Verification items for the finished model (mm, model axes). Face numbers are marked on the shaded views. A direction names the side the tool comes from. Give positions to 0.01 mm unless a question says otherwise; leave off trailing zeros. Write each loop counter-clockwise with the first axis right and the second up, starting at its lowest first coordinate (ties: lowest second). Pieces come first, ordered by that corner, then holes.
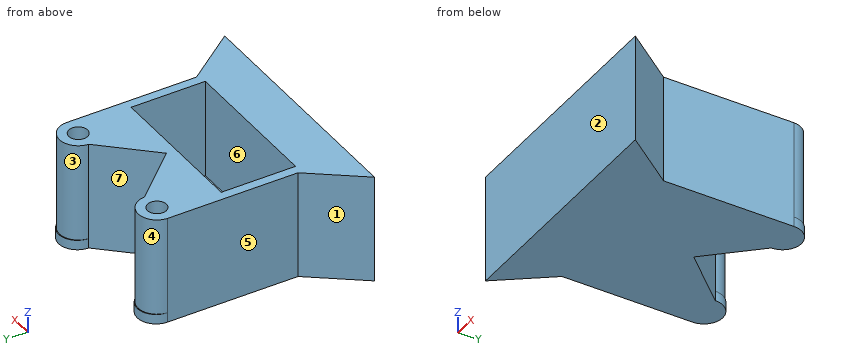
from build123d import *

# Parameters (mm, degrees)
SKETCH1_R           = 4.862500054
SKETCH1_W           = 76.454
SKETCH1_H           = 38.354
BOSS_EXTRUDE1_DEPTH = 50.8
BOSS_EXTRUDE2_DEPTH = 5.08


with BuildPart() as part:
    # Sketch1 → Boss-Extrude1 (new body)
    with BuildSketch(Plane.XY):
        with BuildLine():
            Line((-43.029964919, -17.522331458), (-43.029964919, 19.177))
            Line((-43.029964919, 19.177), (-43.029964919, 49.89109769))
            ThreePointArc((-43.029964919, 49.89109769), (-33.369881409, 59.115507734), (-23.699543278, 49.901848605))
            Line((-23.699543278, 49.901848605), (0, 24.257))
            Line((0, 24.257), (23.699543278, 49.901848605))
            ThreePointArc((23.699543278, 49.901848605), (33.369881409, 59.115507734), (43.029964919, 49.89109769))
            Line((43.029964919, 49.89109769), (43.029964919, 19.177))
            Line((43.029964919, 19.177), (43.029964919, -17.522331458))
            Line((43.029964919, -17.522331458), (63.5, -44.577))
            Line((63.5, -44.577), (-63.5, -44.577))
            Line((-63.5, -44.577), (-43.029964919, -17.522331458))
        make_face()
        with Locations((-33.364499946, 49.439500054)):
            Circle(SKETCH1_R, mode=Mode.SUBTRACT)
        with Locations(Location((33.364499946, 49.439500054, 0), (0, 0, 180))):
            Circle(SKETCH1_R, mode=Mode.SUBTRACT)
        Rectangle(SKETCH1_W, SKETCH1_H, mode=Mode.SUBTRACT)
    extrude(amount=BOSS_EXTRUDE1_DEPTH)

    # Sketch2 → Boss-Extrude2 (add)
    with BuildSketch(Plane(origin=(0, 0, 0), x_dir=(-1, 0, 0), z_dir=(0, 0, -1))):
        with BuildLine():
            Line((-43.029964919, 49.89109769), (-43.029964919, -17.522331458))
            Line((-43.029964919, -17.522331458), (-63.5, -44.577))
            Line((-63.5, -44.577), (63.5, -44.577))
            Line((63.5, -44.577), (43.029964919, -17.522331458))
            Line((43.029964919, -17.522331458), (43.029964919, 49.89109769))
            ThreePointArc((43.029964919, 49.89109769), (33.370126568, 59.556310005), (23.699543278, 49.901848605))
            Line((23.699543278, 49.901848605), (0, 24.257))
            Line((0, 24.257), (-23.699543278, 49.901848605))
            ThreePointArc((-23.699543278, 49.901848605), (-33.370126568, 59.556310005), (-43.029964919, 49.89109769))
        make_face()
    extrude(amount=BOSS_EXTRUDE2_DEPTH)


solid = part.part
Item 1: Sectioned sample at D-D on z = 7.5. Record the cut outline in (x, y) (1 decimal).
Answer key:
outline: (-63.5, -44.6) - (63.5, -44.6) - (43, -17.5) - (43, 49.9) arc R9.7 ccw to (23.7, 49.9) - (0, 24.3) - (-23.7, 49.9) arc R9.7 ccw to (-43, 49.9) - (-43, -17.5) - close; hole (-38.2, -19.2) - (38.2, -19.2) - (38.2, 19.2) - (-38.2, 19.2) - close; hole circle Ø9.7 at (-33.4, 49.4); hole circle Ø9.7 at (33.4, 49.4)
Item 2: Depth check by flat-ended pin: pin 1 (3 mm diameter, centred on y = 39.5, z = 35, fed in from -X); pin 2 (1.5 mm diameter, centred on y = -20, z = 19.5, fed in from -X); pin 3 (6 mm diameter, centred on x = -33.36, y = 49.44, fed in from +Z). Enter the tip coordinate at first touch or a pass-through.
Answer key:
pin 1: stops at x = -43.03
pin 2: stops at x = -45.47
pin 3: stops at z = 0
Item 3: Scan lines: line 1 along Y through (x, z) = (34, 40); line 2 along X through (y, z) = (-8, 8); line 3 along Y through (x, z) = (29, 6). Record each from-to range of solid material in increasing order.
Answer key:
line 1: y = -44.58 to -19.18, 19.18 to 44.62, 54.26 to 59.09
line 2: x = -43.03 to -38.23, 38.23 to 43.03
line 3: y = -44.58 to -19.18, 19.18 to 47.3, 51.58 to 58.08
Item 4: Sectioned sample at C-C on y = 33. Record the cut outline in (x, z).
Answer key:
outline: (-43.03, -5.08) - (-8.08, -5.08) - (-8.08, 50.8) - (-43.03, 50.8) - close; (8.08, -5.08) - (43.03, -5.08) - (43.03, 50.8) - (8.08, 50.8) - close
Item 5: Sectioned sample at B-B on x = -22. Record the cut outline in (y, z).
Answer key:
outline: (-44.58, -5.08) - (48.06, -5.08) - (48.06, 50.8) - (19.18, 50.8) - (19.18, 0) - (-19.18, 0) - (-19.18, 50.8) - (-44.58, 50.8) - close
Item 6: Set-up check for the marked faces 4, 5, 6 and 7: record each of +Z, -Z, +X, -X, +Y, -Y from which the full face is reachable in a straight line by a thin tool's end or side.
Answer key:
face 4: +Z, +Y
face 5: +Z, -Z, -X, +Y
face 6: +Z
face 7: +Z, -Z, +Y
Item 7: Release check for a two-part mould opening along X. For the marked faces 1, 2 and 3 record: released by +X, released by -X, zero draft, split by the parting line, or undercut.
Answer key:
face 1: released by -X
face 2: zero draft
face 3: undercut
Item 8: Sectioned sample at A-A on y = 2. Record the cut outline in (x, z).
Answer key:
outline: (-43.03, -5.08) - (43.03, -5.08) - (43.03, 50.8) - (38.23, 50.8) - (38.23, 0) - (-38.23, 0) - (-38.23, 50.8) - (-43.03, 50.8) - close
